Autodesk Inventor part; units mm, degrees
ref_plane "YZ Plane" through (0, 0, 0) normal (1, 0, 0) x (0, 1, 0)
ref_plane "XZ Plane" through (0, 0, 0) normal (0, 1, 0) x (-1, 0, 0)
ref_plane "XY Plane" through (0, 0, 0) normal (0, 0, 1) x (1, 0, 0)
sketch "Boceto1" plane through (0, 0, 0) normal (0, 1, 0) x (-1, 0, 0)
  arc A0 (-4, -16) -> (4, -16) centre (0, -16) ccw
  arc A1 (4, -2) -> (-4, -2) centre (0, -2) ccw
  line L0 (4, -2) -> (4, -16)
  line L1 (-4, -16) -> (-4, -2)
  line L2 (0, -4) -> (0, -2)
  circle A2 centre (0, -2) radius 1.75
  circle A3 centre (0, -16) radius 1.75
  point P0 (0, 0)
  dimension "d4" = 8
  dimension "d8" = 3.5
  dimension "d9" = 3.5
extrude "Extrusión1" add sketch "Boceto1" along normal blind 3.5 contours L1 A1 L0 A0 | A2 | A3
extrude "Extrusión2" cut sketch "Boceto1" along normal blind 3.5 contours A2 | A3
properties part number "DIREcicon2opala"
The listing builds one solid part. Answer for the finished solid, in the listing's coordinates (mm). Round coordinates to 2 decimals unless told otherwise and drop trailing zeros. Write each loop counter-clockwise with the first axis right and the second up, starting at its lowest first coordinate (ties: lowest second). Pieces come first, ordered by that corner, then holes. Notation, with made-up numbers: (6.25, 82) -> (46.25, 82) arc R26 ccw to (46.25, 112) -> close; hole circle Ø5 at (9, 70.5). An arc over 180 degrees is marked (long way). Use CSV: the item, a comma, the result in double quotes. Start each with the question number.
(1) This flat-tipped pin is pushed along its axis until it touches: pin 1 (2 mm diameter, centred on x = -1, y = 3, fed in from -Z). Where does it stop, or does it pass through?
(2) Consider L1, parallel to Z at x = 0, y = 1.1; L2, parallel to X at y = 1.75, z = -2; L3, parallel to Z at x = 1.5, y = 3. Determine where each line is inside the solid, lowest interval first. Write a range as from..to.
(3) Section D-D on z = -14.75 is taken. Give the vertices of the cut face in (x, y).
(4) The mould has two halves that part along X. Classify faces 1 (the face through (0, 3.5, -9)), 2 (the face through (0, 2, -20)), 3 (the face through (0.38, 1.73, -0.29)): released by +X, released by -X, zero draft, split by the parting line, or undercut.
(5) Section B-B on z = -17 is taken. Give the vertices of the cut face in (x, y), then the cut area to 3 significant figures.
(6) Section C-C on y = 1.5 is taken. Give the vertices of the cut face in (x, z), then the cut area to 3 significant figures.
(7) Section A-A on x = 0 is taken. Give the vertices of the cut face in (y, z), then the cut area to 3 significant figures.
A:
1,pin 1,"stops at z = -20"
2,L1,"z = -20..-17.75, -14.25..-3.75, -0.25..2"
2,L2,"x = -4..-1.75, 1.75..4"
2,L3,"z = -19.71..-16.9, -15.1..-2.9, -1.1..1.71"
3,outline,"(-4, 0) -> (-1.22, 0) -> (-1.22, 3.5) -> (-4, 3.5) -> close; (1.22, 0) -> (4, 0) -> (4, 3.5) -> (1.22, 3.5) -> close"
4,face 1,"zero draft"
4,face 2,"split by the parting line"
4,face 3,"undercut"
5,outline,"(-3.87, 0) -> (-1.44, 0) -> (-1.44, 3.5) -> (-3.87, 3.5) -> close; (1.44, 0) -> (3.87, 0) -> (3.87, 3.5) -> (1.44, 3.5) -> close"
5,area,"17.1 mm²"
6,outline,"(-4, -16) arc R4 ccw to (4, -16) -> (4, -2) arc R4 ccw to (-4, -2) -> close; hole circle Ø3.5 at (0, -16); hole circle Ø3.5 at (0, -2)"
6,area,"143 mm²"
7,outline,"(0, -20) -> (3.5, -20) -> (3.5, -17.75) -> (0, -17.75) -> close; (0, -14.25) -> (3.5, -14.25) -> (3.5, -3.75) -> (0, -3.75) -> close; (0, -0.25) -> (3.5, -0.25) -> (3.5, 2) -> (0, 2) -> close"
7,area,"52.5 mm²"
